Here's how the part is built. I have some questions about the finished solid (model axes, mm). Give positions to 0.01 mm unless a question says otherwise; leave off trailing zeros. Order: outer loops, then holes, each group sorted by start corner. A loop starts at its lowest first (then second) coordinate and runs counter-clockwise, first axis right, second up.
from build123d import *

# Parameters (mm, degrees)
SKETCH_1_R      = 0.4
EXTRUDE_1_DEPTH = 10
SKETCH_2_W      = 80
SKETCH_2_H      = 0.8
EXTRUDE_2_DEPTH = 0.8
FILLET_1_R      = 0.4
SKETCH_3_R      = 0.4
EXTRUDE_3_DEPTH = 3.6
SKETCH_4_R      = 0.4
EXTRUDE_4_DEPTH = 3.6


with BuildPart() as part:
    # 草图1 → 凸台-拉伸1 (new body)
    with BuildSketch(Plane(origin=(0, 0, 0), x_dir=(1, 0, 0), z_dir=(0, 1, 0))):
        with Locations(Location((0, 0, 0), (0, 0, 270))):
            Circle(SKETCH_1_R)
    extrude(amount=EXTRUDE_1_DEPTH)

    # 草图2 → 凸台-拉伸2 (add)
    with BuildSketch(Plane(origin=(0, 10, 0), x_dir=(1, 0, 0), z_dir=(0, 1, 0))):
        Rectangle(SKETCH_2_W, SKETCH_2_H)
    extrude(amount=EXTRUDE_2_DEPTH)

    # 圆角1
    fillet_1_edges = [part.edges().sort_by_distance(p)[0] for p in [
        (40, 10, 0),
        (40, 10.8, 0),
        (-40, 10, 0),
        (-40, 10.8, 0),
    ]]
    fillet(fillet_1_edges, radius=FILLET_1_R - 0.0001)  # a hair under: the kernel refuses the full size

    # 草图3 → 凸台-拉伸3 (add)
    with BuildSketch(Plane.XY.offset(0.4)):
        with Locations((39.6, 10.4)):
            Circle(SKETCH_3_R)
    extrude(amount=EXTRUDE_3_DEPTH)

    # 草图4 → 凸台-拉伸4 (add)
    with BuildSketch(Plane(origin=(0, 0, -0.4), x_dir=(-1, 0, 0), z_dir=(0, 0, -1))):
        with Locations((39.6, 10.4)):
            Circle(SKETCH_4_R)
    extrude(amount=EXTRUDE_4_DEPTH)

    # 草图5 → 旋转1 (revolve)
    with BuildSketch(Plane(origin=(0, 10.4, 0), x_dir=(1, 0, 0), z_dir=(0, 1, 0))):
        Polygon((39.6, -4), (39.6, -5.4), (40, -4), align=None)
    revolve(axis=Axis((39.6, 10.4, 4), (0, 0, 1)))

    # 草图6 → 旋转2 (revolve)
    with BuildSketch(Plane(origin=(0, 10.4, 0), x_dir=(1, 0, 0), z_dir=(0, 1, 0))):
        Polygon((-39.6, 4), (-39.6, 5.4), (-40, 4), align=None)
    revolve(axis=Axis((-39.6, 10.4, -4), (0, 0, -1)))


solid = part.part
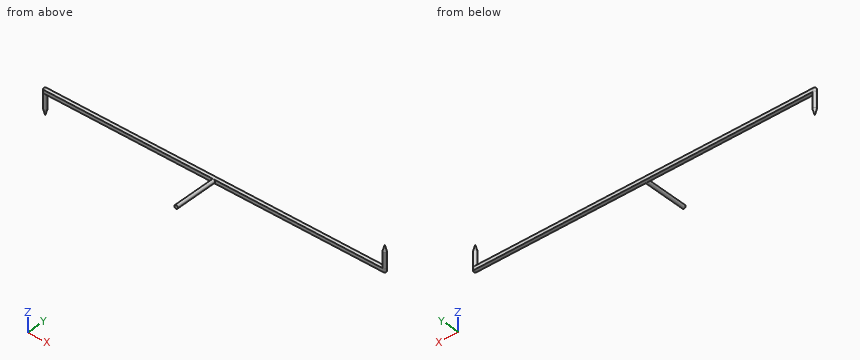
Q1. I'm going to push flat-ended pins straight in: P1, Ø0.6, axis at x = 14, y = 10.5, coming from the -Z side; P2, Ø2, axis at y = 6, z = -1, coming from the +X side; P3, Ø3, axis at y = 9.5, z = 3.5, coming from the +X side; P4, Ø0.9, axis at x = -18.5, z = 0, coming from the -Y side. Where does each tip first touch, or does it pass through?
Filled sheet:
P1: stops at z = -0.4
P2: stops at x = 0.4
P3: stops at x = 40
P4: stops at y = 10
Q2. I need wall thicknesses on L1, parallel to Y at x = 12, z = 0. Which ranges of the line are inside material? Lowest first, please.
Filled sheet:
L1: y = 10 to 10.8
Q3. If we section it at A-A on x = 21: List the corners of the cut face in (y, z) for me.
Filled sheet:
outline: (10, -0.4) - (10.8, -0.4) - (10.8, 0.4) - (10, 0.4) - close
Q4. If we section it at B-B on y = 4.5: List the corners of the cut face in (x, z) for me.
Filled sheet:
outline: circle Ø0.8 at (0, 0)
Q5. If we section it at C-C on z = -2.25: List the corners of the cut face in (x, y) for me.
Filled sheet:
outline: circle Ø0.8 at (-39.6, 10.4)
